Here's the drawing with two shaded views (mm, measured from the low corner). I have some questions. A direction names the side the tool comes from. Round coordinates to 2 decimals unless told otherwise and drop trailing zeros. Write each loop counter-clockwise with the first axis right and the second up, starting at its lowest first coordinate (ties: lowest second). Pieces come first, ordered by that corner, then holes. Notation, with made-up numbers: (-24.75, -37.75) - (13.25, -37.75) arc R18 ccw to (13.25, -14.75) - close; hole circle Ø3 at (-0.75, 10.5). An arc over 180 degrees is marked (long way). Return JSON: item names as keys, results as strings. Group by question number.
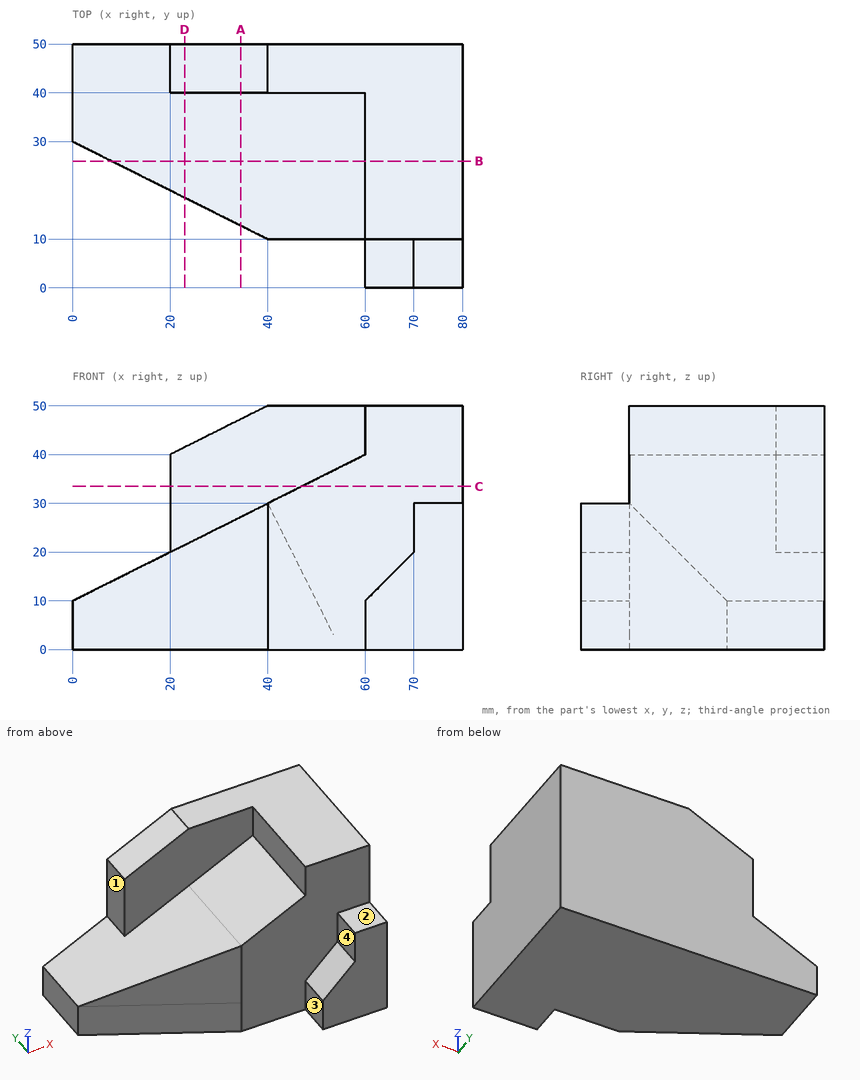
1) I need wall thicknesses on line 1 along Y through (x, z) = (50, 29); line 2 along Y through (x, z) = (54, 43.5); line 3 along X through (y, z) = (3, 3.5). Which ranges of each line are inside material? Lowest first, please.
2) Will these pins go through, and if not, where does the flat tip stop? pin 1 Ø12 at (y, z) = (14.5, 19.5) entering from -X; pin 2 Ø5 at (x, y) = (24, 41) entering from -Z; pin 3 Ø2 at (x, y) = (59.5, 7) entering from +Z; pin 4 Ø9 at (x, z) = (50, 38) entering from -Y.
3) Imagine slicing it at C-C (z = 33.5). Please give me the cut outline in (x, y).
4) Imagine slicing it at A-A (x = 34.5). Please give me the cut outline in (y, z).
5) Imagine slicing it at B-B (y = 26). Please give me the cut outline in (x, z).
6) Imagine slicing it at D-D (x = 23). Please give me the cut outline in (y, z).
7) For the marked faces 1, 2, 3 and 4, which set-ups out of +Z, -Z, +X, -X, +Y, -Y let a thin tool reach every point of the face, with its end or its side?
Results found:
{
 "1": {"line 1": "y = 10 to 50", "line 2": "y = 40 to 50", "line 3": "x = 60 to 80"},
 "2": {"pin 1": "stops at x = 19", "pin 2": "stops at z = 0", "pin 3": "stops at z = 10.5", "pin 4": "stops at y = 10"},
 "3": {"outline": "(20, 40) - (47, 40) - (47, 10) - (80, 10) - (80, 50) - (20, 50) - close"},
 "4": {"outline": "(12.75, 0) - (50, 0) - (50, 47.25) - (40, 47.25) - (40, 27.25) - (12.75, 27.25) - close"},
 "5": {"outline": "(8, 0) - (80, 0) - (80, 50) - (60, 50) - (60, 40) - (8, 14) - close"},
 "6": {"outline": "(18.5, 0) - (50, 0) - (50, 41.5) - (40, 41.5) - (40, 21.5) - (18.5, 21.5) - close"},
 "7": {"face 1": "+Z, -X, +Y, -Y", "face 2": "+Z, +X, -X, -Y", "face 3": "+Z, -Z, -X, -Y", "face 4": "+Z, -X, -Y"}
}
